Check sheet for the modelled part. Datum: model origin and axes. Units: mm. Round coordinates to 2 decimals unless told otherwise and drop trailing zeros. Order: outer loops, then holes, each group sorted by start corner. A loop starts at its lowest first (then second) coordinate and runs counter-clockwise, first axis right, second up. Notation, with made-up numbers: (60, 17) -> (111, 17) arc R21 ccw to (111, 38) -> close; hole circle Ø1 at (-26, -18). An arc over 180 degrees is marked (long way). Answer in a Markdown table with one row per item.
```python
from build123d import *

# Parameters (mm, degrees)
SKETCH2_W  = 12
SKETCH2_H  = 2
SLOT_DEPTH = 3.6


with BuildPart() as part:
    # BodySke → BaseBody (revolve)
    with BuildSketch(Plane.XY, mode=Mode.PRIVATE) as basebody_sk:
        Polygon((50, 0), (50, 4.25), (48.25, 6), (0.556565659, 6), (0, 5.036), (0, 0), align=None)
    revolve(basebody_sk.sketch.rotate(Axis((50, 0, 0), (1, 0, 0)), 90), axis=Axis((50, 0, 0), (1, 0, 0)))

    # Sketch2 → Slot (cut)
    with BuildSketch(Plane(origin=(0, 0, 0), x_dir=(0, 0, -1), z_dir=(1, 0, 0))):
        Rectangle(SKETCH2_W, SKETCH2_H)
    extrude(amount=SLOT_DEPTH, mode=Mode.SUBTRACT)


solid = part.part
```
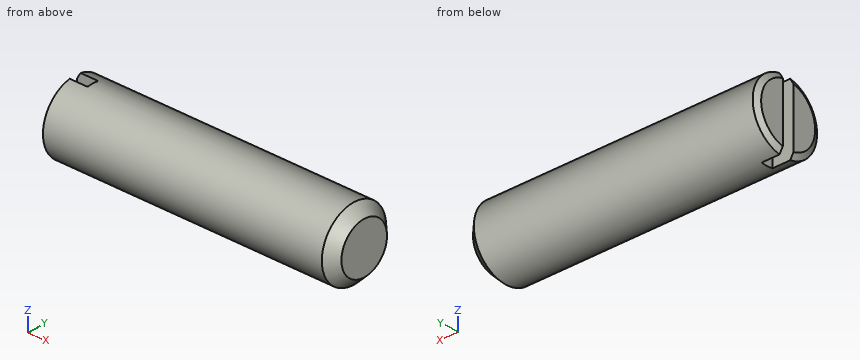
(1) Section check B-B on y = 0. Record the boundary of the cut face in (x, z), plus the area to 3 significant figures.
Solutions:
| item | result |
|---|---|
| outline | (3.6, -6) -> (48.25, -6) -> (50, -4.25) -> (50, 4.25) -> (48.25, 6) -> (3.6, 6) -> close |
| area | 554 mm^2 |
(2) Section check A-A on z = 0. Record the boundary of the cut face in (x, y).
Solutions:
| item | result |
|---|---|
| outline | (0, -5.04) -> (0.56, -6) -> (48.25, -6) -> (50, -4.25) -> (50, 4.25) -> (48.25, 6) -> (0.56, 6) -> (0, 5.04) -> (0, 1) -> (3.6, 1) -> (3.6, -1) -> (0, -1) -> close |
(3) Scan lines: probe 1 along X at (y, z) = (-0.25, -2); probe 2 along Y at (x, z) = (23, -0.25). Record each from-to range of solid material in increasing order. Write a range as from..to.
Solutions:
| item | result |
|---|---|
| probe 1 | 3.6..50 |
| probe 2 | -5.99..5.99 |
(4) Depth check by flat-ended pin: pin 1 Ø3 at (x, y) = (41.5, -1) entering from -Z; pin 2 Ø1.5 at (x, z) = (14, -4.5) entering from -Y; pin 3 Ø4 at (x, y) = (13, 3.5) entering from -Z; pin 4 Ø1.8 at (x, z) = (2, 2.5) entering from +Y. Enter the tip coordinate at first touch or a pass-through.
Solutions:
| item | result |
|---|---|
| pin 1 | z = -6 |
| pin 2 | y = -4.68 |
| pin 3 | z = -5.81 |
| pin 4 | y = 5.78 |
(5) Section check C-C on x = 25. Record the boundary of the cut face in (y, z).
Solutions:
| item | result |
|---|---|
| outline | circle Ø12 at (0, 0) |
